Input: part model. Units: mm. Frame: model coordinates. A direction names the side the tool comes from. Give positions to 0.01 mm unless a question says otherwise; leave off trailing zeros. Order: outer loops, then holes, each group sorted by start corner. A loop starts at its lowest first (then second) coordinate and runs counter-clockwise, first axis right, second up. Notation, with made-up numbers: (-39, 31) - (-12, 31) arc R30 cw to (-12, 62) - close; hole circle Ø1 at (35.25, 13). An arc over 180 degrees is marked (long way). Answer in a Markdown table with one row per item. Add a question column.
1. Section query B-B on y = 33. Return loops of the section in (x, z).
2. Section query D-D on z = -70. Return loops of the section in (x, y).
3. Contact query for flat-ended pins moving along their axis: pin 1 (12 mm diameter, centred on y = 10.5, z = -30, fed in from +X); pin 2 (5 mm diameter, centred on x = 21.5, z = -25, fed in from +Y); pin 3 (10 mm diameter, centred on x = 38.5, z = -108.5, fed in from +Y). Output: stop coordinate, or through.
4. Ray query, line 1 (Z direction, x = 63.5, y = 26); line 2 (X direction, y = 49, z = -7.5). Return the intervals inside material, ascending. Write a range as [from, to].
5. Mould query, pull axis X, two halves, no side actions, for faces 1 (the face through (52.53, 0.373, -21.316)), 2 (the face through (0.373, 19.242, -20.554)), 3 (the face through (1.91, 1.81, -48.59)). Classes: released by +X, released by -X, zero draft, split by the parting line, or undercut.
6. Access query for faces 4 (the face through (56, 29, -142.7)), 5 (the face through (37, 0.737, -53)), 6 (the face through (0.737, 33, -49)), 7 (the face through (0, 33, -49)). Directions: +Z, -Z, +X, -X, +Y, -Y. A direction counts if a zero-diameter tool reaches every point of the face in a straight line with its end or side. Return the directions, or none.
7. Section query C-C on x = 31.5. Return loops of the section in (y, z), and give its area (3 significant figures).
8. Section query A-A on z = -53.34. Return loops of the section in (x, y).
```python
from build123d import *

# Parameters (mm, degrees)
BASE_FLANGE1_DEPTH = 139.7
CUT_EXTRUDE1_START = -139.7
CUT_EXTRUDE1_DEPTH = 41.148
EDGE_FLANGE1_DEPTH = 25.4
FILLET1_RADIUS     = 12.7
FILLET1_LENGTH     = 0.7366
HOLE1_START        = -143.4366
HOLE1_OUTLINE_R    = 4.7625
HOLE1_DEPTH        = 0.7366
SKETCH34_R         = 3.175
CUT_EXTRUDE2_DEPTH = 2.54
SKETCH35_R         = 4.7625
CUT_EXTRUDE3_DEPTH = 2.54
SKETCH36_R         = 3.175
CUT_EXTRUDE4_DEPTH = 2.54


# Read off the part's stored shape, not the designer's step: Cut-Extrude1, Hole1
# Sheet-metal steps are written as plain solids
with BuildPart() as part:
    # Sketch1 → Base-Flange1 (new body)
    with BuildSketch(Plane.XY):
        with BuildLine():
            Line((68.326, 0), (6.35, 0))
            ThreePointArc((6.35, 0), (1.859871939, 1.859871939), (0, 6.35))
            Line((0, 6.35), (0, 59.881871389))
            ThreePointArc((0, 59.881871389), (1.415123145, 63.878055872), (5.029760763, 66.093108654))
            Line((5.029760763, 66.093108654), (42.926, 74.148202966))
            Line((42.926, 74.148202966), (43.079147751, 73.427699444))
            Line((43.079147751, 73.427699444), (5.182908515, 65.372605131))
            ThreePointArc((5.182908515, 65.372605131), (1.98756886, 63.414498472), (0.7366, 59.881871389))
            Line((0.7366, 59.881871389), (0.7366, 6.35))
            ThreePointArc((0.7366, 6.35), (2.380726794, 2.380726794), (6.35, 0.7366))
            Line((6.35, 0.7366), (68.326, 0.7366))
            Line((68.326, 0.7366), (68.326, 0))
        make_face()
    extrude(amount=-BASE_FLANGE1_DEPTH)

    # Cut-Extrude1 outline → Cut-Extrude1 (cut)
    with BuildSketch(Plane.XY.offset(CUT_EXTRUDE1_START)):
        with BuildLine():
            Line((6.35, 0), (42.926, 0))
            Line((42.926, 0), (42.926, 0.7366))
            Line((42.926, 0.7366), (6.35, 0.7366))
            ThreePointArc((6.35, 0.7366), (2.380726794, 2.380726794), (0.7366, 6.35))
            Line((0.7366, 6.35), (0.7366, 59.881871389))
            ThreePointArc((0.7366, 59.881871389), (1.98756886, 63.414498472), (5.182908515, 65.372605131))
            Line((5.182908515, 65.372605131), (43.079147751, 73.427699444))
            Line((43.079147751, 73.427699444), (42.926, 74.148202966))
            Line((42.926, 74.148202966), (5.029760763, 66.093108654))
            ThreePointArc((5.029760763, 66.093108654), (1.415123145, 63.878055872), (0, 59.881871389))
            Line((0, 59.881871389), (0, 6.35))
            ThreePointArc((0, 6.35), (1.859871939, 1.859871939), (6.35, 0))
        make_face()
    extrude(amount=CUT_EXTRUDE1_DEPTH, mode=Mode.SUBTRACT)

    # Edge-Flange1 section (across the edge) → Edge-Flange1 (add)
    with BuildSketch(Plane(origin=(68.326, 0.7366, -142.7), x_dir=(0, 0, 1), z_dir=(-1, 0, 0))):
        with BuildLine():
            Line((-0.7366, 3), (-0.7366, 52.6034))
            Line((-0.7366, 52.6034), (0, 52.6034))
            Line((0, 52.6034), (0, 3))
            ThreePointArc((0, 3), (0.878679656, 0.878679656), (3, 0))
            Line((3, 0), (3, -0.7366))
            ThreePointArc((3, -0.7366), (0.357824801, 0.357824801), (-0.7366, 3))
        make_face()
    extrude(amount=EDGE_FLANGE1_DEPTH)

    # Fillet1: full round fillet: the end face becomes a half cylinder, R = half its width
    fillet1_face = Plane((55.626, 53.34, -143.0683), x_dir=(0, 0, -1), z_dir=(0, 1, 0))  # on the end face: x along it, z out of the body
    fillet1_slab = fillet1_face.offset(-FILLET1_RADIUS / 2) * Box(FILLET1_LENGTH, 2 * FILLET1_RADIUS, FILLET1_RADIUS, mode=Mode.PRIVATE)  # the body's end, R deep
    fillet1_round = Plane((55.626, 40.64, -143.0683), x_dir=(0, 1, 0), z_dir=(0, 0, -1)) * Cylinder(FILLET1_RADIUS, FILLET1_LENGTH, mode=Mode.PRIVATE)  # its axis R under the face
    add(fillet1_slab - fillet1_round, mode=Mode.SUBTRACT)

    # Hole1 outline → Hole1 (cut)
    with BuildSketch(Plane.XY.offset(HOLE1_START)):
        with Locations((55.626, 40.64)):
            Circle(HOLE1_OUTLINE_R)
    extrude(amount=HOLE1_DEPTH, mode=Mode.SUBTRACT)

    # Sketch34 → Cut-Extrude2 (cut)
    with BuildSketch(Plane(origin=(-13.22382174, 62.213189919, 0), x_dir=(0.9781476007338064, 0.20791169081775657, 0), z_dir=(-0.20791169081775657, 0.9781476007338064, 0))):
        with Locations(Location((35.814242159, 19.05, 0), (0, 0, 180))):
            Circle(SKETCH34_R)
        with Locations(Location((35.814242159, 82.55, 0), (0, 0, 180))):
            Circle(SKETCH34_R)
    extrude(amount=-CUT_EXTRUDE2_DEPTH, mode=Mode.SUBTRACT)

    # Sketch35 → Cut-Extrude3 (cut)
    with BuildSketch(Plane(origin=(0, 0.7366, 0), x_dir=(1, 0, 0), z_dir=(0, 1, 0))):
        with Locations(Location((48.514, 23.876, 0), (0, 0, 270))):
            Circle(SKETCH35_R)
        with Locations(Location((48.514, 53.34, 0), (0, 0, 270))):
            Circle(SKETCH35_R)
    extrude(amount=-CUT_EXTRUDE3_DEPTH, mode=Mode.SUBTRACT)

    # Sketch36 → Cut-Extrude4 (cut)
    with BuildSketch(Plane(origin=(0.7366, 0, 0), x_dir=(0, 0, -1), z_dir=(1, 0, 0))):
        with Locations((17.526, 18.288)):
            Circle(SKETCH36_R)
        with Locations((75.438, 18.288)):
            Circle(SKETCH36_R)
        with Locations((17.526, 47.752)):
            Circle(SKETCH36_R)
        with Locations((75.438, 47.752)):
            Circle(SKETCH36_R)
    extrude(amount=-CUT_EXTRUDE4_DEPTH, mode=Mode.SUBTRACT)


solid = part.part
```
Answer:
| question | item | result |
|---|---|---|
| 1 | outline | (0, -98.55) - (0.74, -98.55) - (0.74, 0) - (0, 0) - close; (42.93, -143.44) - (68.33, -143.44) - (68.33, -142.7) - (42.93, -142.7) - close |
| 2 | outline | (0, 6.35) arc R6.35 ccw to (6.35, 0) - (68.33, 0) - (68.33, 0.74) - (6.35, 0.74) arc R5.61 cw to (0.74, 6.35) - (0.74, 59.88) arc R5.61 cw to (5.18, 65.37) - (43.08, 73.43) - (42.93, 74.15) - (5.03, 66.09) arc R6.35 ccw to (0, 59.88) - close |
| 3 | pin 1 | stops at x = 1.05 |
| 3 | pin 2 | stops at y = 70.13 |
| 3 | pin 3 | stops at y = 0.74 |
| 4 | line 1 | z = [-143.44, -142.7] |
| 4 | line 2 | x = [0, 0.74] |
| 5 | face 1 | undercut |
| 5 | face 2 | zero draft |
| 5 | face 3 | released by -X |
| 6 | face 4 | +Z, +X, -X, +Y |
| 6 | face 5 | +Z, +X |
| 6 | face 6 | +Z, -Z, +X |
| 6 | face 7 | +Z, -Z, -X, +Y, -Y |
| 7 | outline | (0, -98.55) - (0.74, -98.55) - (0.74, 0) - (0, 0) - close; (70.97, -98.55) - (71.72, -98.55) - (71.72, 0) - (70.97, 0) - close |
| 7 | area | 147 mm² |
| 8 | outline | (0, 6.35) arc R6.35 ccw to (6.35, 0) - (43.75, 0) - (43.75, 0.74) - (6.35, 0.74) arc R5.61 cw to (0.74, 6.35) - (0.74, 59.88) arc R5.61 cw to (5.18, 65.37) - (43.08, 73.43) - (42.93, 74.15) - (5.03, 66.09) arc R6.35 ccw to (0, 59.88) - close; (53.28, 0) - (68.33, 0) - (68.33, 0.74) - (53.28, 0.74) - close |
